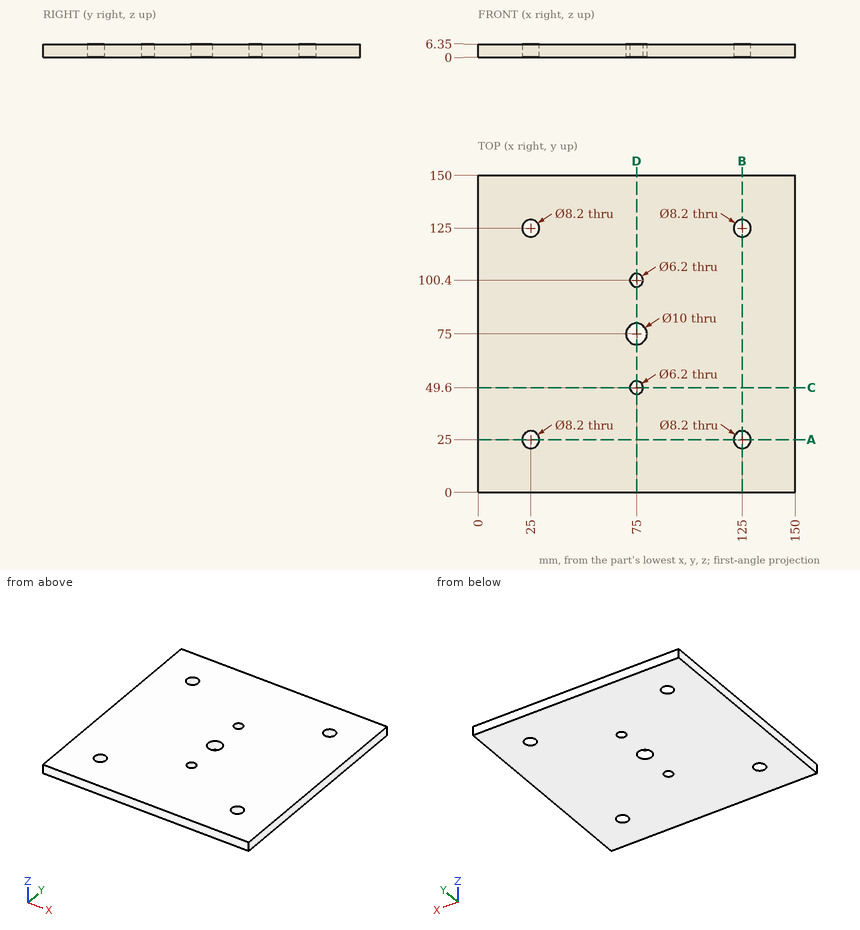
Design review of the part shown in the three views and the two pictorial views. Dimensions are in mm from the part's minimum x, y and z. Give positions to 0.01 mm unless a question says otherwise; leave off trailing zeros. Write each loop counter-clockwise with the first axis right and the second up, starting at its lowest first coordinate (ties: lowest second). Pieces come first, ordered by that corner, then holes.
(1) Add section A-A (y = 25). Give the boundary of the cut face in (x, z), and give its area (3 significant figures).
Checked values:
outline: (0, 0) - (20.9, 0) - (20.9, 6.35) - (0, 6.35) - close; (29.1, 0) - (120.9, 0) - (120.9, 6.35) - (29.1, 6.35) - close; (129.1, 0) - (150, 0) - (150, 6.35) - (129.1, 6.35) - close
area: 848 mm2
(2) Wall thickness on line 1 along Y through (x, z) = (25, 2); line 2 along Y through (x, z) = (124, 0.5); line 3 along X through (y, z) = (76, 2.5): over which ranges is each line inside the solid? List them lowest first.
Checked values:
line 1: y = 0 to 20.9, 29.1 to 120.9, 129.1 to 150
line 2: y = 0 to 21.02, 28.98 to 121.02, 128.98 to 150
line 3: x = 0 to 70.1, 79.9 to 150
(3) Clearance check with a flat-ended pin moving along its axis: pin 1 Ø7.5 at (x, y) = (125, 125) entering from +Z. State where the tip first meets the part, or that it passes through.
Checked values:
pin 1: passes through
(4) Add section C-C (y = 49.6). Give the boundary of the cut face in (x, z), and give its area (3 significant figures).
Checked values:
outline: (0, 0) - (71.9, 0) - (71.9, 6.35) - (0, 6.35) - close; (78.1, 0) - (150, 0) - (150, 6.35) - (78.1, 6.35) - close
area: 913 mm2
(5) Add section D-D (x = 75). Give the boundary of the cut face in (y, z).
Checked values:
outline: (0, 0) - (46.5, 0) - (46.5, 6.35) - (0, 6.35) - close; (52.7, 0) - (70, 0) - (70, 6.35) - (52.7, 6.35) - close; (80, 0) - (97.3, 0) - (97.3, 6.35) - (80, 6.35) - close; (103.5, 0) - (150, 0) - (150, 6.35) - (103.5, 6.35) - close
